Job drawing, mm, ordinate dimensions from the low corner. One solid piece. Coordinates: 2 decimals unless noted, no trailing zeros. Write each loop counter-clockwise with the first axis right and the second up, starting at its lowest first coordinate (ties: lowest second). Pieces come first, ordered by that corner, then holes. Notation, with made-up numbers: (37.5, 5.5) -> (77.5, 5.5) arc R12 cw to (77.5, 21.5) -> close; hole circle Ø3 at (27, 34.25). An arc over 180 degrees is marked (long way). One line per question, with ' | ' between items. Start each with the question number.
Item 1: Saw through at D-D (y = 0.85). Count the separate pieces of the cut face and the enclosed holes in it, and give its area (3 significant figures).
Item 2: Saw through at A-A (z = 21.5). List the corners of the cut face in (x, y) (3 decimals).
Item 3: Probe probe 1 along X at (y, z) = (1.6, 25); probe 2 along X at (y, z) = (1.2, 50); probe 3 along X at (y, z) = (1.4, 70). List the from-to ranges inside material, lowest first. Write a range as [from, to].
Item 4: Pin check, flat tip, straight feed: pin 1 (1 mm diameter, centred on y = 1, z = 125.5, fed in from -X). Stop position of the tip, or through.
Item 5: Saw through at C-C (z = 122.5). List the corners of the cut face in (x, y) (3 decimals), and give its area (3 significant figures).
Item 6: Saw through at B-B (x = 187). List the corners of the cut face in (y, z) (3 decimals), and give its area (4 significant figures).
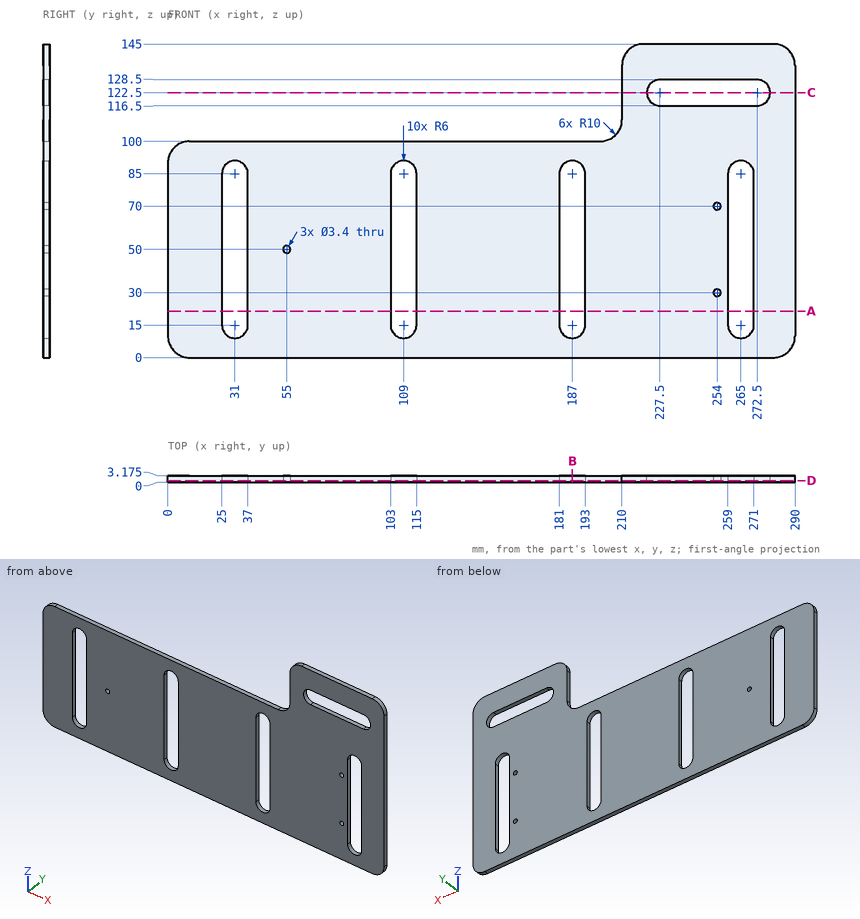
From the geometry:
1) separate pieces: 1 | enclosed holes: 8 | area: 28,000 mm2
2) outline: (0, 0) -> (25, 0) -> (25, 3.175) -> (0, 3.175) -> close; (37, 0) -> (103, 0) -> (103, 3.175) -> (37, 3.175) -> close; (115, 0) -> (181, 0) -> (181, 3.175) -> (115, 3.175) -> close; (193, 0) -> (259, 0) -> (259, 3.175) -> (193, 3.175) -> close; (271, 0) -> (290, 0) -> (290, 3.175) -> (271, 3.175) -> close
3) probe 1: [0, 25], [37, 103], [115, 181], [193, 259], [271, 290] | probe 2: [0, 25], [37, 53.3], [56.7, 103], [115, 181], [193, 259], [271, 290] | probe 3: [0, 25], [37, 103], [115, 181], [193, 252.3], [255.7, 259], [271, 290]
4) pin 1: x = 210
5) outline: (210, 0) -> (221.5, 0) -> (221.5, 3.175) -> (210, 3.175) -> close; (278.5, 0) -> (290, 0) -> (290, 3.175) -> (278.5, 3.175) -> close | area: 73.0 mm2
6) outline: (0, 0) -> (3.175, 0) -> (3.175, 9) -> (0, 9) -> close; (0, 91) -> (3.175, 91) -> (3.175, 100) -> (0, 100) -> close | area: 57.15 mm2
